```python
from build123d import *

# Parameters (mm, degrees)
BOSS_EXTRUDE1_DEPTH                          = 1
CSK_FOR_M3_COUNTERSUNK_FLAT_HEAD_SCR_2_COUNT = 2
CSK_FOR_M3_COUNTERSUNK_FLAT_HEAD_SCR_2_PITCH = 34.11906313
CSK_FOR_M3_COUNTERSUNK_FLAT_HEAD_SCR_3_COUNT = 2
CSK_FOR_M3_COUNTERSUNK_FLAT_HEAD_SCR_3_PITCH = 24.08237255
CSK_FOR_M3_COUNTERSUNK_FLAT_HEAD_SCR_4_COUNT = 2
CSK_FOR_M3_COUNTERSUNK_FLAT_HEAD_SCR_4_PITCH = 24.085156004
BOSS_EXTRUDE3_DEPTH                          = 5.5
FILLET1_R                                    = 2
FILLET2_R                                    = 1


with BuildPart() as part:
    # Sketch5 → Boss-Extrude1 (new body)
    with BuildSketch(Plane(origin=(0, 0, 0), x_dir=(1, 0, 0), z_dir=(0, 1, 0))):
        with BuildLine():
            Line((-18.02, 12.02), (-18.02, -12.02))
            ThreePointArc((-18.02, -12.02), (-16.262640687, -16.262640687), (-12.02, -18.02))
            Line((-12.02, -18.02), (12.02, -18.02))
            ThreePointArc((12.02, -18.02), (16.262640687, -16.262640687), (18.02, -12.02))
            Line((18.02, -12.02), (18.02, 12.02))
            ThreePointArc((18.02, 12.02), (16.262640687, 16.262640687), (12.02, 18.02))
            Line((12.02, 18.02), (-12.02, 18.02))
            ThreePointArc((-12.02, 18.02), (-16.262640687, 16.262640687), (-18.02, 12.02))
        make_face()
    extrude(amount=-BOSS_EXTRUDE1_DEPTH)

    # Sketch15 → CSK for M3 Countersunk Flat Head Screw3 (revolve, cut)
    with BuildSketch(Plane(origin=(-12.037863248, 0, 12.033949607), x_dir=(0, 0, 1), z_dir=(1, 0, 0))):
        Polygon((0, 0), (0, 1.001), (1.7, 1.001), (1.7, 1.45), (3.15, 0), align=None)
    csk_for_m3_countersunk_flat_head_screw3 = revolve(axis=Axis((-12.037863248, 6.35, 12.033949607), (0, -1, 0)), mode=Mode.SUBTRACT)

    # CSK for M3 Countersunk Flat Head Scr 2: CSK for M3 Countersunk Flat Head Screw3 ×2
    with Locations(*[Vector(0.706351229, 0, -0.707861527) * (i * CSK_FOR_M3_COUNTERSUNK_FLAT_HEAD_SCR_2_PITCH) for i in range(1, CSK_FOR_M3_COUNTERSUNK_FLAT_HEAD_SCR_2_COUNT)]):
        add(csk_for_m3_countersunk_flat_head_screw3, mode=Mode.SUBTRACT)

    # CSK for M3 Countersunk Flat Head Scr 3: CSK for M3 Countersunk Flat Head Screw3 ×2
    with Locations(*[(i * CSK_FOR_M3_COUNTERSUNK_FLAT_HEAD_SCR_3_PITCH, 0, 0) for i in range(1, CSK_FOR_M3_COUNTERSUNK_FLAT_HEAD_SCR_3_COUNT)]):
        add(csk_for_m3_countersunk_flat_head_screw3, mode=Mode.SUBTRACT)

    # CSK for M3 Countersunk Flat Head Scr 4: CSK for M3 Countersunk Flat Head Screw3 ×2
    with Locations(*[Vector(-0.000330161, 0, -0.999999945) * (i * CSK_FOR_M3_COUNTERSUNK_FLAT_HEAD_SCR_4_PITCH) for i in range(1, CSK_FOR_M3_COUNTERSUNK_FLAT_HEAD_SCR_4_COUNT)]):
        add(csk_for_m3_countersunk_flat_head_screw3, mode=Mode.SUBTRACT)

    # Sketch16 → Boss-Extrude3 (add)
    with BuildSketch(Plane.XZ.offset(1)):
        with BuildLine():
            Line((18.02, -12.02), (18.02, 12.02))
            ThreePointArc((18.02, 12.02), (16.262640687, 16.262640687), (12.02, 18.02))
            Line((12.02, 18.02), (-12.02, 18.02))
            ThreePointArc((-12.02, 18.02), (-16.262640687, 16.262640687), (-18.02, 12.02))
            Line((-18.02, 12.02), (-18.02, -12.02))
            ThreePointArc((-18.02, -12.02), (-16.262640687, -16.262640687), (-12.02, -18.02))
            Line((-12.02, -18.02), (12.02, -18.02))
            ThreePointArc((12.02, -18.02), (16.262640687, -16.262640687), (18.02, -12.02))
        make_face()
        with BuildLine():
            Line((17.02, -12.02), (17.02, 12.02))
            ThreePointArc((17.02, 12.02), (15.555533906, 15.555533906), (12.02, 17.02))
            Line((12.02, 17.02), (-12.02, 17.02))
            ThreePointArc((-12.02, 17.02), (-15.555533906, 15.555533906), (-17.02, 12.02))
            Line((-17.02, 12.02), (-17.02, -12.02))
            ThreePointArc((-17.02, -12.02), (-15.555533906, -15.555533906), (-12.02, -17.02))
            Line((-12.02, -17.02), (12.02, -17.02))
            ThreePointArc((12.02, -17.02), (15.555533906, -15.555533906), (17.02, -12.02))
        make_face(mode=Mode.SUBTRACT)
    extrude(amount=BOSS_EXTRUDE3_DEPTH)

    # Fillet1
    fillet1_edges = [part.edges().sort_by_distance(p)[0] for p in [
        (16.262640687, 0, 16.262640687),
        (0, 0, 18.02),
        (-16.262640687, 0, 16.262640687),
        (-18.02, 0, 0),
        (-16.262640687, 0, -16.262640687),
        (0, 0, -18.02),
        (16.262640687, 0, -16.262640687),
        (18.02, 0, 0),
    ]]
    fillet(fillet1_edges, radius=FILLET1_R)

    # Fillet2
    fillet2_edges = [part.edges().sort_by_distance(p)[0] for p in [
        (15.555533906, -1, -15.555533906),
        (17.02, -1, 0),
        (15.555533906, -1, 15.555533906),
        (0, -1, 17.02),
        (-15.555533906, -1, 15.555533906),
        (-17.02, -1, 0),
        (-15.555533906, -1, -15.555533906),
        (0, -1, -17.02),
    ]]
    fillet(fillet2_edges, radius=FILLET2_R)


solid = part.part
```
Here's how the part is built. I have some questions about the finished solid (model axes, mm). A direction names the side the tool comes from. Coordinates: 2 decimals unless noted, no trailing zeros. Order: outer loops, then holes, each group sorted by start corner. A loop starts at its lowest first (then second) coordinate and runs counter-clockwise, first axis right, second up.
1) Which directions (+Z, -Z, +X, -X, +Y, -Y) give clear straight access to the entire face, cutting with the end or side of a thin tool? Please do faces 4 (the face through (-17.02, -4, 0)), 5 (the face through (18.02, -4, 0)).
2) Imagine slicing it at D-D on z = 12.5. State how many separate pieces and enclosed holes the cut face has, and give its area (3 significant figures).
3) Will this pin go through, and if not, where does the flat tip stop? pin 1 (3 mm diameter, centred on x = -8.5, z = 12, fed in from -Y).
4) We'd pull the mould along Z, two halves only. Please class faces 1 (the face through (-0.1, -6.5, -17.3)), 2 (the face through (-0.168, -1.301, 16.735)), 3 (the face through (0.17, -0.57, 17.42)): +Z half, -Z half, draft (parallel to the pull), parting line (faces both ways), or undercut.
5) Imagine slicing it at C-C on z = 6.5. List the corners of the cut face in (x, y) for me, and give its area (3 significant figures).
6) Imagine slicing it at A-A on x = 7. List the corners of the cut face in (y, z) for me.
7) Imagine slicing it at B-B on y = -4.5. List the corners of the cut face in (x, z) for me.
8) I need wall thicknesses on line 1 (Z direction, x = 9, y = -5); line 2 (Y direction, x = -8.5, z = -7). Which ranges of each line are inside material? Lowest first, please.
Response values:
1. face 4: -Y
1. face 5: +Z, -Z, +X, +Y, -Y
2. separate pieces: 3
2. enclosed holes: 0
2. area: 35.3 mm2
3. pin 1: stops at y = -1
4. face 1: draft
4. face 2: undercut
4. face 3: +Z half
5. outline: (-18.02, -6.5) - (-17.02, -6.5) - (-17.02, -2) arc R1 cw to (-16.02, -1) - (16.02, -1) arc R1 cw to (17.02, -2) - (17.02, -6.5) - (18.02, -6.5) - (18.02, -2) arc R2 ccw to (16.02, 0) - (-16.02, 0) arc R2 ccw to (-18.02, -2) - close
5. area: 45.8 mm2
6. outline: (-6.5, -18.02) - (-2, -18.02) arc R2 ccw to (0, -16.02) - (0, 16.02) arc R2 ccw to (-2, 18.02) - (-6.5, 18.02) - (-6.5, 17.02) - (-2, 17.02) arc R1 cw to (-1, 16.02) - (-1, -16.02) arc R1 cw to (-2, -17.02) - (-6.5, -17.02) - close
7. outline: (-18.02, -12.02) arc R6 ccw to (-12.02, -18.02) - (12.02, -18.02) arc R6 ccw to (18.02, -12.02) - (18.02, 12.02) arc R6 ccw to (12.02, 18.02) - (-12.02, 18.02) arc R6 ccw to (-18.02, 12.02) - close; hole (-17.02, -12.02) arc R5 ccw to (-12.02, -17.02) - (12.02, -17.02) arc R5 ccw to (17.02, -12.02) - (17.02, 12.02) arc R5 ccw to (12.02, 17.02) - (-12.02, 17.02) arc R5 ccw to (-17.02, 12.02) - close
8. line 1: z = -18.02 to -17.02, 17.02 to 18.02
8. line 2: y = -1 to 0
